Source: CAD feature listing. Evaluate the final solid. Frame: model axes, mm. Face numbers are marked on the shaded views. A direction names the side the tool comes from. Round coordinates to 2 decimals unless told otherwise and drop trailing zeros. Order: outer loops, then holes, each group sorted by start corner. A loop starts at its lowest first (then second) coordinate and runs counter-clockwise, first axis right, second up. Notation, with made-up numbers: (89.5, 41) -> (101.5, 41) arc R34 cw to (101.5, 77) -> close; hole circle Ø8 at (56, 89.25). An arc over 180 degrees is marked (long way). Use a Markdown table: item, result. Add a question column.
Autodesk Fusion 360 part; units mm, degrees
sketch "Sketch1" plane through (0, 0, 0) normal (0, 0, 1) x (1, 0, 0)
  line L0 (36, 27) -> (-36, 27)
  line L1 (-36, 27) -> (-36, -27)
  line L2 (-36, -27) -> (36, -27)
  line L3 (36, -27) -> (36, 27)
  line L4 (36, 30.6) -> (-36, 30.6)
  line L5 (-36, 35.6) -> (-36, -30.6)
  line L6 (-36, -30.6) -> (36, -30.6)
  line L7 (36, -30.6) -> (36, 30.6)
  line L8 (33, 35.6) -> (-36, 35.6)
  line L9 (41, -27.6) -> (41, 27.6)
  line L10 (33, -35.6) -> (-36, -35.6)
  line L11 (-36, -35.6) -> (-36, 30.6)
  arc A0 (41, 27.6) -> (33, 35.6) centre (33, 27.6) ccw
  arc A1 (33, -35.6) -> (41, -27.6) centre (33, -27.6) ccw
  circle A2 centre (-20, 0) radius 1.75
  line L12 (-19.9571, 11) -> (-5, 11)
  arc A3 (-5, 11) -> (-5, 19) centre (-5, 15) ccw
  line L13 (-5, 19) -> (-19.9571, 19)
  arc A4 (-19.9571, 19) -> (-19.9571, 11) centre (-19.9571, 15) ccw
  line L14 (-19.9571, 15) -> (-5, 15) construction
  line L15 (1.75, 0) -> (22.5, 0)
  line L16 (-19.9571, -11) -> (-5, -11)
  line L17 (-5, -19) -> (-19.9571, -19)
  arc A5 (-5, -19) -> (-5, -11) centre (-5, -15) ccw
  arc A6 (-19.9571, -11) -> (-19.9571, -19) centre (-19.9571, -15) ccw
  circle A7 centre (-5, 0) radius 1.75
  dimension "d1" = 72
  dimension "d2" = 54
  dimension "d3" = 61.2
  dimension "d6" = 8
  dimension "d32" = 3.5
  dimension "d34" = 8
  dimension "d40" = 3.5
extrude "Extrude1" add sketch "Sketch1" along normal blind 6.3 contours L3 L4 L5 L6 L7 L8 L9 L10 L11 A0 A1 | L0 L4 L5 L7 L11 | L2 L5 L6 L7 L11
extrude "Extrude2" add sketch "Sketch1" along normal blind 24 contours L3 L4 L5 L6 L7 L8 L9 L10 L11 A0 A1
extrude "Extrude3" add sketch "Sketch1" along normal blind 27 and the other way blind -24
sketch "Sketch2" plane through (0, -35.6, 0) normal (0, -1, 0) x (1, 0, 0)
  line L0 (-36, 0) -> (33, 0)
  line L1 (33, 0) -> (33, 27)
  line L2 (-36, 27) -> (-36, 0)
  line L3 (-36, 0) -> (-49.5029, 27)
  line L4 (-36, 0) -> (-6, 0) construction
  line L5 (-36, 27) -> (-49.5029, 27)
  line L6 (33, 27) -> (-36, 27)
  line L7 (-36, 27) -> (-36, 24)
  line L8 (-36, 24) -> (-36.4845, 24)
  line L9 (-36.4845, 24) -> (-48.0026, 24)
  line L10 (-36, 0) -> (-36, 6.4)
  line L11 (-36, 6.4) -> (-36, 6)
  line L12 (-36, 6.4) -> (-39.2007, 6.4)
  line L13 (-36, 0) -> (-32.4, 0)
  line L14 (-49.5029, 27) -> (-47.5029, 27)
  line L15 (-36, 6.4) -> (-32.4, 6.4)
  line L16 (-32.4, 6.4) -> (-32.4, 0)
  dimension "d11" = 116.57
  dimension "d25" = 6.4
  dimension "d36" = 3.6
  dimension "d37" = 2
extrude "Extrude4" add sketch "Sketch2" against normal blind 5 contours L2 L3 L10 L11 L12 | L2 L3 L8 L9 L12
extrude "Extrude5" add sketch "Sketch2" along normal blind -71.2 and the other way blind 66.2 contours L2 L3 L10 L11 L12 | L2 L3 L8 L9 L12
extrude "Extrude6" add sketch "Sketch2" against normal blind 71.2 contours L2 L3 L5 L7 L8 L9 L14
extrude "Extrude7" cut sketch "Sketch2" along normal blind -8.6 and the other way blind 5 contours L0 L2 L10 L11 L13 L15 L16
extrude "Extrude8" cut sketch "Sketch2" along normal blind -66.2 and the other way blind 62.6 contours L0 L2 L10 L11 L13 L15 L16
chamfer "Chamfer2" distance 1 angle 45 2 edges at (-21.6316, 0.6328, 24) (-6.6316, 0.6328, 24)
sketch "Sketch3" plane through (0, 0, 27) normal (0, 0, 1) x (-1, 0, 0)
  arc A0 (5, 19) -> (5, 11) centre (5, 15) ccw
  line L0 (5, 19) -> (19.9571, 19)
  arc A1 (19.9571, 11) -> (19.9571, 19) centre (19.9571, 15) ccw
  line L1 (19.9571, 11) -> (5, 11)
  circle A2 centre (20, 0) radius 1.75
  circle A3 centre (5, 0) radius 1.75
  arc A4 (19.9571, -19) -> (19.9571, -11) centre (19.9571, -15) ccw
  line L2 (19.9571, -19) -> (5, -19)
  arc A5 (5, -11) -> (5, -19) centre (5, -15) ccw
  line L3 (5, -11) -> (19.9571, -11)
  line L4 (49.5029, 35.6) -> (-33, 35.6)
  arc A6 (-33, 35.6) -> (-41, 27.6) centre (-33, 27.6) ccw
  line L5 (-41, 27.6) -> (-41, -27.6)
  arc A7 (-41, -27.6) -> (-33, -35.6) centre (-33, -27.6) ccw
  line L6 (-33, -35.6) -> (49.5029, -35.6)
  line L7 (49.5029, -35.6) -> (49.5029, 35.6)
  line L8 (-5, -40) -> (-45, -40)
  line L9 (-45, -40) -> (-45, 40)
  line L10 (-45, 40) -> (-5, 40)
  line L11 (-5, 40) -> (-5, -40)
extrude "Extrude9" cut sketch "Sketch3" against normal blind 55 contours L4 A6 L5 A7 L6 L11 | L4 A6 L5 A7 L6 L8 L9 L10 L11
chamfer "Chamfer3" distance 1 angle 45 2 edges at (-32.4, -28.8, 6.3) (-32.4, 28.8, 6.3)
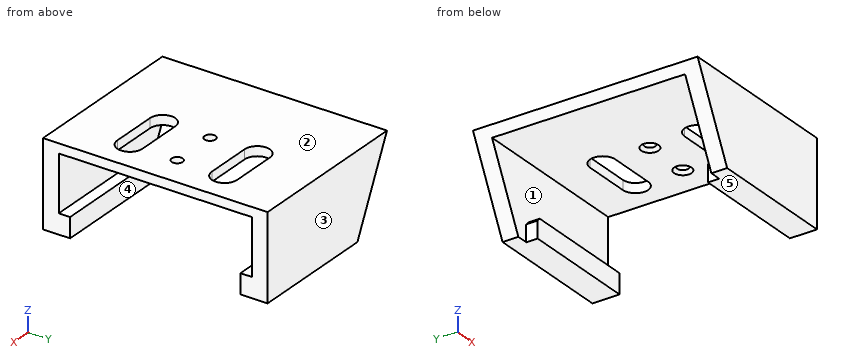
1) Section A-A on z = 8. Output: boundary loops of the cut face in (x, y).
2) Section B-B on y = -15. Output: boundary loops of the cut face in (x, z), then the cut area to 3 significant figures.
3) Reachability of the marked faces 4 and 5 from +Z, -Z, +X, -X, +Y, -Y: full face, straight path, thin tool, end or side. Return the list, or none.
4) Line query: probe 1 along Y at (x, z) = (-20, 25.7); probe 2 along Y at (x, z) = (-39, 21.5); probe 3 along Z at (x, y) = (-24, -28). Output: solid intervals per line, ascending. Write a range as from..to.
5) Section D-D on z = 4.25. Output: boundary loops of the cut face in (x, y), then the cut area to 3 significant figures.
6) Section C-C on x = -39. Output: boundary loops of the cut face in (y, z).
7) Draft query along Z for the marked faces 1, 2 and 3. Return one class per face: pulls with the +Z half, pulls with the -Z half, needs draft (parallel to the pull), parting line crosses it, or undercut.
8) First-contact query: pin 1 Ø4 at (y, z) = (-29.5, 3.5) entering from -X; pin 2 Ø3 at (y, z) = (28.5, 16.5) entering from -X; pin 3 Ø1.8 at (y, z) = (28, 2.5) entering from -X; pin 4 Ø3 at (x, y) = (-8.5, -22.5) entering from -Z. Flat tips, straight axial feed; report the tip coordinate or a pass-through.
Conclusion:
| question | item | result |
|---|---|---|
| 1 | outline | (-40, -35.6) -> (5, -35.6) -> (5, -30.6) -> (-40, -30.6) -> close; (-40, 30.6) -> (5, 30.6) -> (5, 35.6) -> (-40, 35.6) -> close |
| 2 | outline | (-49.5, 27) -> (-48, 24) -> (-23.96, 24) -> (-23.96, 27) -> close; (-1, 24) -> (5, 24) -> (5, 27) -> (-1, 27) -> close |
| 2 | area | 92.4 mm^2 |
| 3 | face 4 | -Z, +X, -X |
| 3 | face 5 | -Z, +X, -X, +Y, -Y |
| 4 | probe 1 | y = -35.6..-19, -11..-1.75, 1.75..11, 19..35.6 |
| 4 | probe 2 | y = -35.6..-30.6, 30.6..35.6 |
| 4 | probe 3 | z = 0..6.3, 24..27 |
| 5 | outline | (-38.13, -35.6) -> (5, -35.6) -> (5, -27) -> (-32.4, -27) -> (-32.4, -30.6) -> (-38.13, -30.6) -> close; (-38.13, 30.6) -> (-32.4, 30.6) -> (-32.4, 27) -> (5, 27) -> (5, 35.6) -> (-38.13, 35.6) -> close |
| 5 | area | 701 mm^2 |
| 6 | outline | (-35.6, 6) -> (-30.6, 6) -> (-30.6, 24) -> (30.6, 24) -> (30.6, 6) -> (35.6, 6) -> (35.6, 27) -> (-35.6, 27) -> close |
| 7 | face 1 | undercut |
| 7 | face 2 | pulls with the +Z half |
| 7 | face 3 | needs draft |
| 8 | pin 1 | stops at x = -38.59 |
| 8 | pin 2 | passes through |
| 8 | pin 3 | stops at x = -32.4 |
| 8 | pin 4 | stops at z = 24 |
